from build123d import *

# Parameters (mm, degrees)
BOSS_EXTRUDE1_DEPTH = 7
SKETCH2_R           = 10
CUT_EXTRUDE1_DEPTH  = 8


with BuildPart() as part:
    # Sketch1 → Boss-Extrude1 (new body)
    with BuildSketch(Plane(origin=(0, 0, 0), x_dir=(0, 0, -1), z_dir=(1, 0, 0))):
        Polygon((-7, -31), (-7, -45), (7, -45), (7, -31), (17.5, -31), (17.5, 31), (7, 31), (7, 45), (-7, 45), (-7, 31), (-17.5, 31), (-17.5, -31), align=None)
    extrude(amount=BOSS_EXTRUDE1_DEPTH)

    # Sketch2 → Cut-Extrude1 (cut, through all)
    with BuildSketch(Plane(origin=(7, 0, 0), x_dir=(0, 0, -1), z_dir=(1, 0, 0))):
        Circle(SKETCH2_R)
    extrude(amount=-CUT_EXTRUDE1_DEPTH, mode=Mode.SUBTRACT)


solid = part.part
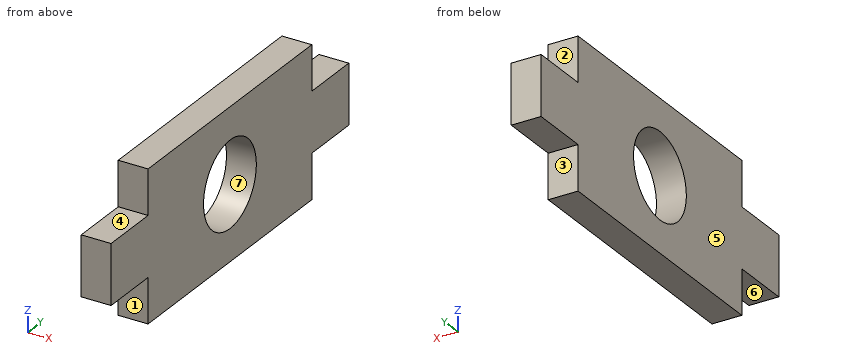
Geometry check sheet. Reference: the model listing, model coordinates, mm. Face numbers are marked on the shaded views. A direction names the side the tool comes from. Coordinates: 2 decimals unless noted, no trailing zeros. Order: outer loops, then holes, each group sorted by start corner. A loop starts at its lowest first (then second) coordinate and runs counter-clockwise, first axis right, second up. Notation, with made-up numbers: (51, 19) - (59, 19) arc R5 cw to (59, 23) - close; hole circle Ø11 at (87.25, 23). An arc over 180 degrees is marked (long way). One line per item, written item: value.
(1) Release check for a two-part mould opening along Z. For the marked faces 5, 6 and 7 record: +Z half, -Z half, draft (parallel to the pull), parting line (faces both ways), or undercut.
Data:
face 5: draft
face 6: -Z half
face 7: undercut
(2) Sectioned sample at B-B (x = 3). Enter the section's corners in (y, z), and give its area (3 significant figures).
Data:
outline: (-45, -7) - (-31, -7) - (-31, -17.5) - (31, -17.5) - (31, -7) - (45, -7) - (45, 7) - (31, 7) - (31, 17.5) - (-31, 17.5) - (-31, 7) - (-45, 7) - close; hole circle Ø20 at (0, 0)
area: 2,250 mm^2
(3) Sectioned sample at C-C (y = 0). Enter the section's corners in (x, z), and give its area (3 significant figures).
Data:
outline: (0, -17.5) - (7, -17.5) - (7, -10) - (0, -10) - close; (0, 10) - (7, 10) - (7, 17.5) - (0, 17.5) - close
area: 105 mm^2
(4) Sectioned sample at D-D (y = -35.5). Enter the section's corners in (x, z).
Data:
outline: (0, -7) - (7, -7) - (7, 7) - (0, 7) - close
(5) Access from +Z, -Z, +X, -X, +Y, -Y to the whole of each face (thin tool, end or side, straight path). Record for the marked faces 1, 2, 3 and 4.
Data:
face 1: -Z, +X, -X, -Y
face 2: +Z, +X, -X, +Y
face 3: -Z, +X, -X, +Y
face 4: +Z, +X, -X, -Y
(6) Thickness scan on probe 1 along Y at (x, z) = (1.5, 0); probe 2 along Y at (x, z) = (4.75, 11.5); probe 3 along Z at (x, y) = (5, 32.5). Record the ranges inside material, lowest first. Write a range as from..to.
Data:
probe 1: y = -45..-10, 10..45
probe 2: y = -31..31
probe 3: z = -7..7
(7) Depth check by flat-ended pin: pin 1 Ø2 at (x, y) = (2, 36) entering from +Z; pin 2 Ø2 at (x, y) = (3.5, 39.5) entering from -Z; pin 3 Ø2 at (x, z) = (2.5, -12) entering from +Y. Enter the tip coordinate at first touch or a pass-through.
Data:
pin 1: stops at z = 7
pin 2: stops at z = -7
pin 3: stops at y = 31
(8) Sectioned sample at A-A (z = 0). Enter the section's corners in (x, y).
Data:
outline: (0, -45) - (7, -45) - (7, -10) - (0, -10) - close; (0, 10) - (7, 10) - (7, 45) - (0, 45) - close
